from build123d import *

# Parameters (mm, degrees)
SKETCH2_R           = 1
BOSS_EXTRUDE1_DEPTH = 1
CUT_EXTRUDE1_START  = 1
SKETCH3_R           = 2.75
CUT_EXTRUDE1_DEPTH  = 0.6


with BuildPart() as part:
    # Sketch2 → Boss-Extrude1 (new body)
    with BuildSketch(Plane.XY):
        Polygon((16.46, 48.53), (32.57, 32.53), (73.99, 32.53), (94.6, 53.03), (73.99, 73.53), (32.57, 73.53), (16.46, 57.53), (12.07, 57.53), (12.07, 48.53), align=None)
        with Locations((24.5, 59.53)):
            Circle(SKETCH2_R, mode=Mode.SUBTRACT)
        with Locations((24.5, 46.53)):
            Circle(SKETCH2_R, mode=Mode.SUBTRACT)
        with Locations((83, 60.03)):
            Circle(SKETCH2_R, mode=Mode.SUBTRACT)
        with Locations((83, 46.03)):
            Circle(SKETCH2_R, mode=Mode.SUBTRACT)
    extrude(amount=BOSS_EXTRUDE1_DEPTH)

    # Sketch3 → Cut-Extrude1 (cut)
    with BuildSketch(Plane.XY.offset(CUT_EXTRUDE1_START)):
        with Locations((24.5, 59.53)):
            Circle(SKETCH3_R)
        with Locations((24.5, 46.53)):
            Circle(SKETCH3_R)
        with Locations((83, 60.03)):
            Circle(SKETCH3_R)
        with Locations((83, 46.03)):
            Circle(SKETCH3_R)
    extrude(amount=-CUT_EXTRUDE1_DEPTH, mode=Mode.SUBTRACT)


solid = part.part
Could you check a few things on this model? Use its own coordinates, in mm. A direction names the side the tool comes from. Round coordinates to 2 decimals unless told otherwise and drop trailing zeros. Write each loop counter-clockwise with the first axis right and the second up, starting at its lowest first coordinate (ties: lowest second). Pieces come first, ordered by that corner, then holes. Notation, with made-up numbers: (39.25, 21) - (67.25, 21) arc R27 cw to (67.25, 47) - close; hole circle Ø2 at (43, -4). An arc over 180 degrees is marked (long way). Put each result on its own line as item: value. Start each with the question number.
(1) I want a section at A-A, the plane x = 24.5. Please give me the cut outline in (y, z).
(2) Will these pins go through, and if not, where does the flat tip stop? pin 1 (3.5 mm diameter, centred on x = 24.5, y = 59.53, fed in from +Z); pin 2 (0.5 mm diameter, centred on x = 14.5, z = 0.5, fed in from -Y).
(3) Thinking about a two-plate mould opening in Y: for faces 3 (the cylindrical face through (82, 60.07, 0.2)), 4 (the flat face through (84.151, 42.636, 0.493)), 5 (the flat face through (53, 53, 0)), which applies, released by +Y, released by -Y, zero draft, split by the parting line, or undercut?
(4) I want a section at C-C, the plane y = 40. Please give me the cut outline in (x, z), plus the area to 3 significant figures.
(5) I want a section at B-B, the plane x = 83. Please give me the cut outline in (y, z), plus the area to 3 significant figures.
(6) I need wall thicknesses on probe 1 along Y at (x, z) = (83, 0.6); probe 2 along X at (y, z) = (59.53, 0.25); probe 3 along X at (y, z) = (60.03, 0.3). Which ranges of each line are inside material? Lowest first, please.
(7) For faces 1 (the flat face through (24, 45, 0.4)), 2 (the flat face through (24.402, 40.642, 0.493)), which set-ups out of +Z, -Z, +X, -X, +Y, -Y let a thin tool reach every point of the face, with its end or its side?
Here are the results:
1. outline: (40.54, 0) - (45.53, 0) - (45.53, 0.4) - (43.78, 0.4) - (43.78, 1) - (40.54, 1) - close; (47.53, 0) - (58.53, 0) - (58.53, 0.4) - (56.78, 0.4) - (56.78, 1) - (49.28, 1) - (49.28, 0.4) - (47.53, 0.4) - close; (60.53, 0) - (65.52, 0) - (65.52, 1) - (62.28, 1) - (62.28, 0.4) - (60.53, 0.4) - close
2. pin 1: stops at z = 0.4
2. pin 2: stops at y = 48.53
3. face 3: undercut
3. face 4: released by -Y
3. face 5: zero draft
4. outline: (25.05, 0) - (81.5, 0) - (81.5, 1) - (25.05, 1) - close
4. area: 56.5 mm^2
5. outline: (41.49, 0) - (45.03, 0) - (45.03, 0.4) - (43.28, 0.4) - (43.28, 1) - (41.49, 1) - close; (47.03, 0) - (59.03, 0) - (59.03, 0.4) - (57.28, 0.4) - (57.28, 1) - (48.78, 1) - (48.78, 0.4) - (47.03, 0.4) - close; (61.03, 0) - (64.57, 0) - (64.57, 1) - (62.78, 1) - (62.78, 0.4) - (61.03, 0.4) - close
5. area: 14.9 mm^2
6. probe 1: y = 41.49 to 43.28, 48.78 to 57.28, 62.78 to 64.57
6. probe 2: x = 18.47 to 23.5, 25.5 to 82.13, 83.87 to 88.07
6. probe 3: x = 18.98 to 23.63, 25.37 to 82, 84 to 87.56
7. face 1: +Z
7. face 2: +Z, -Z, -X, -Y
